Design review of the part built by this model. Coordinates are the model's own, in mm. Face numbers are marked on the shaded views. A direction names the side the tool comes from. Give positions to 0.01 mm unless a question says otherwise; leave off trailing zeros. Loops run counter-clockwise (first coordinate to the right, second up) from the corner with the lowest first, then second, coordinate; pieces in that order, holes last. Notation, with made-up numbers: M -30.5,-11.5 L 17.5,-11.5 A27 ccw 17.5,25.5 Z; hole C 14,-19 d8. An arc over 180 degrees is marked long. Use a Markdown table: item, result. Add a question column.
(1) Add section D-D, the plane z = -20. Give the boundary of the cut face in (x, y).
(2) Draft analysis for pull direction X (two halves, no side actions). For the marked faces 1, 2, 3 and 4, state which applies: pulls with the +X half, pulls with the -X half, needs draft (parallel to the pull), parting line crosses it, or undercut.
(3) Add section A-A, the plane z = 0. State how many separate pieces and enclosed holes the cut face has, then the cut area to 3 significant figures.
(4) Add section B-B, the plane x = 0. Give the boundary of the cut face in (y, z).
(5) Insertion check: pin 1 Ø15 at (x, y) = (-49.5, 6) entering from +Z; pin 2 Ø1.5 at (y, z) = (1, 21) entering from +X; pin 3 Ø8 at (x, z) = (-30.5, 9.5) entering from +Y. Each pin has a flat end and moves straight along its axis. Give the tip position at first contact, or say it passes through.
(6) For probe 1 along Y at (x, z) = (55, 11); probe 2 along X at (y, z) = (-5.25, -10); probe 3 along X at (y, z) = (2, -16), list the stretches that pass through material, from the lowest coordinate up.
(7) For the marked faces 5, 6 and 7, list the 3-axis set-ups (+Z, -Z, +X, -X, +Y, -Y) from which the entire face can be reached by the end or side of a thin tool; tool diameter is ignored.
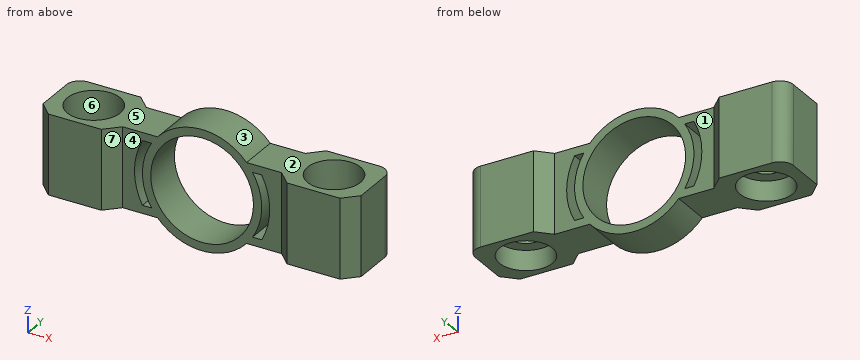
```python
from build123d import *

# Parameters (mm, degrees)
SKETCH1_W             = 36
SKETCH1_H             = 36
BOSS_EXTRUDE3_DEPTH   = 15
BOSS_EXTRUDE3_2_DEPTH = 15
SKETCH1_6_R           = 23.25
BOSS_EXTRUDE4_DEPTH   = 9
CHAMFER3_SIZE         = 6
FILLET1_R             = 6
SKETCH2_R             = 6.5
CUT_EXTRUDE2_DEPTH    = 64.5
SKETCH2_4_R           = 12
SKETCH2_4_R_2         = 6.5
CUT_EXTRUDE3_DEPTH    = 19.5
CUT_EXTRUDE5_START    = -7.5
SKETCH4_R             = 12
SKETCH4_R_2           = 6.5
CUT_EXTRUDE5_DEPTH    = 87


with BuildPart() as part:
    # Sketch1 → Boss-Extrude3 (new, symmetric)
    with BuildSketch(Plane(origin=(0, 0, 0), x_dir=(1, 0, 0), z_dir=(0, 1, 0))):
        with Locations((-54, 0)):
            Rectangle(SKETCH1_W, SKETCH1_H)
    extrude(amount=BOSS_EXTRUDE3_DEPTH, both=True)



with BuildPart() as body_2:
    # Sketch1 → Boss-Extrude3 2 (new, symmetric)
    with BuildSketch(Plane(origin=(0, 0, 0), x_dir=(1, 0, 0), z_dir=(0, 1, 0))):
        with Locations((54, 0)):
            Rectangle(SKETCH1_W, SKETCH1_H)
    extrude(amount=BOSS_EXTRUDE3_2_DEPTH, both=True)


with BuildPart() as part_1:
    add(part.part)

    add(body_2.part)  # Boss-Extrude4 merges body 2
    # Sketch1<6> → Boss-Extrude4 (add, symmetric)
    with BuildSketch(Plane(origin=(0, 0, 0), x_dir=(1, 0, 0), z_dir=(0, 1, 0))):
        with BuildLine():
            Line((-72, -18), (-20.124611797, -18))
            ThreePointArc((-20.124611797, -18), (0, -27), (20.124611797, -18))
            Line((20.124611797, -18), (72, -18))
            Line((72, -18), (72, 18))
            Line((72, 18), (20.124611797, 18))
            ThreePointArc((20.124611797, 18), (0, 27), (-20.124611797, 18))
            Line((-20.124611797, 18), (-72, 18))
            Line((-72, 18), (-72, -18))
        make_face()
        with Locations(Location((0, 0, 0), (0, 0, 270))):
            Circle(SKETCH1_6_R, mode=Mode.SUBTRACT)
        with BuildLine():
            Line((22.839439573, 14.4), (27, 14.4))
            ThreePointArc((27, 14.4), (30.6, 0), (27, -14.4))
            Line((27, -14.4), (22.839439573, -14.4))
            ThreePointArc((22.839439573, -14.4), (27, 0), (22.839439573, 14.4))
        make_face(mode=Mode.SUBTRACT)
        with BuildLine():
            Line((-27, 14.4), (-22.839439573, 14.4))
            ThreePointArc((-22.839439573, 14.4), (-27, 0), (-22.839439573, -14.4))
            Line((-22.839439573, -14.4), (-27, -14.4))
            ThreePointArc((-27, -14.4), (-30.6, 0), (-27, 14.4))
        make_face(mode=Mode.SUBTRACT)
    extrude(amount=BOSS_EXTRUDE4_DEPTH, both=True)

    # Chamfer3
    chamfer3_edges = [part_1.edges().sort_by_distance(p)[0] for p in [
        (36, 15, 0),
        (72, -15, 0),
        (36, -15, 0),
        (-36, -15, 0),
        (-72, -15, 0),
        (-36, 15, 0),
    ]]
    chamfer(chamfer3_edges, length=CHAMFER3_SIZE - 0.0001)  # a hair under: the kernel refuses the full size

    # Fillet1
    fillet1_edges = [part_1.edges().sort_by_distance(p)[0] for p in [
        (-72, 15, 0),
        (72, 15, 0),
    ]]
    fillet(fillet1_edges, radius=FILLET1_R)

    # Sketch2 → Cut-Extrude2 (cut)
    with BuildSketch(Plane.XY.offset(18)):
        with Locations((-54.369879574, 0)):
            Circle(SKETCH2_R)
        with Locations((54.369879574, 0)):
            Circle(SKETCH2_R)
    extrude(amount=-CUT_EXTRUDE2_DEPTH, mode=Mode.SUBTRACT)

    # Sketch2<4> → Cut-Extrude3 (cut)
    # profile 1 of 2: a face of its own
    with BuildSketch(Plane.XY.offset(18)):
        with Locations((-54.369879574, 0)):
            Circle(SKETCH2_4_R)
        with Locations((-54.369879574, 0)):
            Circle(SKETCH2_4_R_2, mode=Mode.SUBTRACT)
    # profile 2 of 2: a face of its own
    with BuildSketch(Plane.XY.offset(18)):
        with Locations(Location((54.369879574, 0, 0), (0, 0, 180))):
            Circle(SKETCH2_4_R)
        with Locations((54.369879574, 0)):
            Circle(SKETCH2_4_R_2, mode=Mode.SUBTRACT)
    extrude(amount=-CUT_EXTRUDE3_DEPTH, mode=Mode.SUBTRACT)

    # Sketch4 → Cut-Extrude5 (cut)
    # profile 1 of 2: a face of its own
    with BuildSketch(Plane.XY.offset(-1.5).offset(CUT_EXTRUDE5_START)):
        with Locations(Location((54.369879574, 0, 0), (0, 0, 180))):
            Circle(SKETCH4_R)
        with Locations((54.369879574, 0)):
            Circle(SKETCH4_R_2, mode=Mode.SUBTRACT)
    # profile 2 of 2: a face of its own
    with BuildSketch(Plane.XY.offset(-1.5).offset(CUT_EXTRUDE5_START)):
        with Locations((-54.369879574, 0)):
            Circle(SKETCH4_R)
        with Locations((-54.369879574, 0)):
            Circle(SKETCH4_R_2, mode=Mode.SUBTRACT)
    extrude(amount=-CUT_EXTRUDE5_DEPTH, mode=Mode.SUBTRACT)


solid = part_1.part
```
Established:
| question | item | result |
|---|---|---|
| 1 | outline | M -18.14,-9 L -11.86,-9 L -11.86,9 L -18.14,9 Z; M 11.86,-9 L 18.14,-9 L 18.14,9 L 11.86,9 Z |
| 2 | face 1 | undercut |
| 2 | face 2 | needs draft |
| 2 | face 3 | parting line crosses it |
| 2 | face 4 | undercut |
| 3 | separate pieces | 4 |
| 3 | enclosed holes | 2 |
| 3 | area | 1,460 mm^2 |
| 4 | outline | M -9,-27 L 9,-27 L 9,-23.25 L -9,-23.25 Z; M -9,23.25 L 9,23.25 L 9,27 L -9,27 Z |
| 5 | pin 1 | z = 18 |
| 5 | pin 2 | x = 17.86 |
| 5 | pin 3 | y = 9 |
| 6 | probe 1 | -15 to -11.98, 11.98 to 15 |
| 6 | probe 2 | -72 to -65.16, -43.58 to -28.92, -25.08 to -20.99, 20.99 to 25.08, 28.92 to 43.58, 65.16 to 72 |
| 6 | probe 3 | -72 to -66.2, -42.54 to -16.87, 16.87 to 42.54, 66.2 to 72 |
| 7 | face 5 | +Z, -X, +Y, -Y |
| 7 | face 6 | +Z |
| 7 | face 7 | +Z, -Z, -Y |
